Work out the finished part from the listing and answer in its coordinate system (mm). A direction names the side the tool comes from. Round coordinates to 2 decimals unless told otherwise and drop trailing zeros. Write each loop counter-clockwise with the first axis right and the second up, starting at its lowest first coordinate (ties: lowest second). Pieces come first, ordered by that corner, then holes. Notation, with made-up numbers: M 65,26.5 L 118,26.5 A20 ccw 118,52.5 Z; hole C -28.5,58.5 d6. An arc over 180 degrees is marked long. One line per item, written item: value. Start each with the question number.
Q1. Find section B-B (y = 1). Write down the section's boundary in (x, z).
Q2. Find section A-A (x = -20). Write down the section's boundary in (y, z).
Q3. Consider probe 1 along X at (y, z) = (-1.1, 16.5); probe 2 along Z at (x, y) = (32, 2.25). Determine where each line is inside the solid, lowest interval first.
Q4. The mould has two halves that part along X. Classify faces 3 (the flat face through (1, 0, 28.119)), 4 (the flat face through (72.889, 0, -1)), 5 (the flat face through (-1, 0, -39.723)): released by +X, released by -X, zero draft, split by the parting line, or undercut.
Q5. Find section C-C (z = -7). Write down the section's boundary in (x, y), and give its area (3 significant figures).
Q6. A tool of negligible diameter and unlimited length cuts with its end or side. For faces 1 (the flat face through (-1, -2.5, -26)), 2 (the flat face through (-36.506, 0, 2)), from which of +Z, -Z, +X, -X, +Y, -Y can it reach the whole face along a straight path? Write none if from no direction.
from build123d import *

# Parameters (mm, degrees)
F0_W     = 145.778776
F0_H     = 79.445884
F0_W_2   = 75.186506
F0_H_2   = 52.17734
F1_DEPTH = 2.5


with BuildPart() as f1:
    # F0 (on Front) → F1 (new body, symmetric)
    with BuildSketch(Plane.XZ):
        Rectangle(F0_W, F0_H)
        with Locations((1.087524, 2.030745)):
            Rectangle(F0_W_2, F0_H_2, mode=Mode.SUBTRACT)
    extrude(amount=F1_DEPTH, both=True)


solid = f1.part
The answers:
1. outline: M -72.89,-39.72 L 72.89,-39.72 L 72.89,39.72 L -72.89,39.72 Z; hole M -36.51,-24.06 L 38.68,-24.06 L 38.68,28.12 L -36.51,28.12 Z
2. outline: M -2.5,-39.72 L 2.5,-39.72 L 2.5,-24.06 L -2.5,-24.06 Z; M -2.5,28.12 L 2.5,28.12 L 2.5,39.72 L -2.5,39.72 Z
3. probe 1: -72.89 to -36.51, 38.68 to 72.89
3. probe 2: -39.72 to -24.06, 28.12 to 39.72
4. face 3: undercut
4. face 4: released by +X
4. face 5: zero draft
5. outline: M -72.89,-2.5 L -36.51,-2.5 L -36.51,2.5 L -72.89,2.5 Z; M 38.68,-2.5 L 72.89,-2.5 L 72.89,2.5 L 38.68,2.5 Z
5. area: 353 mm2
6. face 1: +Z, -Z, +X, -X, -Y
6. face 2: +Y, -Y
